Autodesk Inventor part; units mm, degrees
ref_plane "YZ Plane" through (0, 0, 0) normal (1, 0, 0) x (0, 1, 0)
ref_plane "XZ Plane" through (0, 0, 0) normal (0, 1, 0) x (-1, 0, 0)
ref_plane "XY Plane" through (0, 0, 0) normal (0, 0, 1) x (1, 0, 0)
ref_plane "Plano de trabajo1" through (0, 0, 0) normal (0, 0, 1) x (1, 0, 0)
sketch "Boceto1" plane through (0, 0, 0) normal (0, 0, 1) x (1, 0, 0)
  circle A0 centre (18.3423, 0) radius 1.2028
  circle A1 centre (3.6423, 0) radius 1.2028
  circle A2 centre (10.9923, -7.35) radius 1.2028
  circle A3 centre (10.9923, 7.35) radius 1.2028
  circle A4 centre (10.9923, 0) radius 10.9823
  circle A5 centre (10.9923, 0) radius 2.7
  circle A6 centre (10.9923, 0) radius 12.5
  line L0 (10.9923, 0) -> (22.9923, 0)
  line L1 (10.9923, 0) -> (10.9923, 12.5)
  line L2 (10.9923, 12.5) -> (22.9923, 12.5)
  line L3 (10.9923, 0) -> (10.9923, -12.5)
  line L4 (10.9923, -12.5) -> (22.9923, -12.5)
  line L5 (22.9923, -12.5) -> (22.9923, 12.5)
  point P0 (0, 0)
  dimension "d0" = 25
  dimension "d1" = 12
  dimension "d2" = 12
extrude "Extrusión1" add sketch "Boceto1" along normal blind 3 contours L0 A4 L3 A2 A5 A0 | A0 L0 A5 L1 A3 A4 | L0 L5 A6 L3 A4 | A4 L1 A6 L5 L0 | L1 A3 A5 L3 A2 A4 | A4 L3 A6 L1 | L2 L5 A6 | A6 L5 L4
sketch "Boceto2" plane through (22.9923, -12.5, 0) normal (1, 0, 0) x (0, 0, -1)
  line L0 (0, 0) -> (0, 25)
  line L1 (0, 25) -> (-3, 25)
  line L2 (-3, 0) -> (-3, 25)
  line L3 (0, 0) -> (-3, 0)
  point P0 (0, 12.5)
extrude "Extrusión2" add sketch "Boceto2" along normal blind 8
sketch "Boceto3" plane through (0, 0, 0) normal (0, 0, -1) x (-1, 0, 0)
  line L0 (-10.9923, -12.5) -> (-30.9923, -12.5)
  arc A0 (-10.9923, -12.5) -> (-10.9923, 12.5) centre (-10.9923, 0) ccw
  line L1 (-10.9923, 12.5) -> (-30.9923, 12.5)
  line L2 (-30.9923, -12.5) -> (-30.9923, 12.5)
  circle A1 centre (-10.9923, 0) radius 2.7
  circle A2 centre (-10.9923, 7.35) radius 1.2028
  circle A3 centre (-18.3423, 0) radius 1.2028
  circle A4 centre (-3.6423, 0) radius 1.2028
  circle A5 centre (-10.9923, -7.35) radius 1.2028
  line L3 (-30.9923, 12.5) -> (-27.9923, 12.5)
  line L4 (-27.9923, 12.5) -> (-27.9923, -12.5)
  line L5 (-27.9923, -12.5) -> (-30.9923, -12.5)
  line L6 (-30.9923, -12.5) -> (-30.9923, 12.5)
  point P0 (0, 0)
  dimension "d7" = 3
extrude "Extrusión3" add sketch "Boceto3" along normal blind 42 contours L0 L2 L1 L4
sketch "Boceto4" plane through (27.9923, -12.5, 0) normal (-1, 0, 0) x (0, 0, 1)
  line L0 (-42, 0) -> (-42, 25)
  line L1 (0, 25) -> (0, 0)
  line L2 (0, 25) -> (-42, 25)
  line L3 (-42, 0) -> (-42, 25)
  line L4 (0, 0) -> (-42, 0)
  line L5 (-42, 0) -> (-40, 0)
  line L6 (-40, 0) -> (-40, 25)
  line L7 (-40, 25) -> (-42, 25)
  line L8 (-42, 25) -> (-42, 0)
  point P0 (0, 12.5)
  dimension "d10" = 2
extrude "Extrusión4" add sketch "Boceto4" along normal blind 30 contours L0 L2 L6 L4
sketch "Boceto5" plane through (0, 0, -42) normal (0, 0, -1) x (-1, 0, 0)
  line L0 (24.4501, 12.6367) -> (24.5578, -12.3277)
  line L1 (-11.0672, 12.4835) -> (24.4501, 12.6367)
  arc A0 (-11.0672, 12.4835) -> (-10.9596, -12.4809) centre (-11.0134, 0.0013) ccw
  line L2 (-10.9596, -12.4809) -> (24.5578, -12.3277)
  circle A1 centre (-3.6676, 0.2495) radius 1.2028
  circle A2 centre (-11.0134, 0.0013) radius 2.7
  circle A3 centre (-10.7652, -7.3445) radius 1.2028
  circle A4 centre (-11.2616, 7.3471) radius 1.2028
  circle A5 centre (-18.3592, -0.2469) radius 1.2028
  line L3 (-30.9923, 12.5) -> (2.0077, 12.5)
  line L4 (-11.0672, 12.4835) -> (2.0077, 12.5)
  line L5 (2.0391, -12.4248) -> (2.0077, 12.5)
  line L6 (-10.9596, -12.4809) -> (2.0391, -12.4248)
  line L7 (-11.0672, 12.4835) -> (2.0077, 12.5)
  circle A6 centre (-11.0134, 0.0013) radius 12.4823
  line L8 (-10.7652, -7.3445) -> (-10.7652, -14.8497)
  line L9 (-10.7652, -14.8497) -> (6.2045, -14.8497)
  line L10 (6.2045, -14.8497) -> (6.2045, 15.7882)
  line L11 (6.2045, 15.7882) -> (-10.7652, 15.7882)
  line L12 (-10.7652, 15.7882) -> (-11.2616, 7.3471)
  point P0 (0, 0)
  point P1 (-7.2489, 12.5)
  point P2 (-10.991, 12.4836)
  point P3 (-10.9817, -12.481)
  point P4 (-10.9586, 12.5)
  point P5 (6.2045, 12.558)
  point P6 (6.2045, -12.4069)
  point P7 (-10.7652, -12.48)
  point P8 (-10.9595, 12.484)
  point P9 (-10.9595, 12.4837)
  point P10 (-10.9596, 12.4835)
  point P11 (-10.991, 12.4836)
  point P12 (-10.7652, -12.4785)
  point P13 (-11.0672, 12.4835)
extrude "Extrusión5" cut sketch "Boceto5" against normal blind 25 contours L10 L2 L5 L3 L1 | L1 L3 L12 L11 L10 | L10 L9 L8 L2 | L3 L4 L1 | L1 L12 L3 | L2 A6 L4 L5 | A3 | A4 | A1 | A2 | A5
sketch "Boceto8" plane through (10.9923, -12.5, 0) normal (0, -1, 0) x (1, 0, 0)
  line L0 (-0.2271, -40) -> (-0.2271, -42)
  line L1 (20, -42) -> (-0.2271, -42)
  line L2 (20, 3) -> (20, -42)
  line L3 (0, 3) -> (20, 3)
  line L4 (0, 0) -> (0, 3)
  line L5 (0, 0) -> (17, 0)
  line L6 (17, 0) -> (17, -40)
  line L7 (17, -40) -> (-0.2271, -40)
  line L8 (20, -42) -> (20, -19.5)
  line L9 (20, 3) -> (20, -42)
  line L10 (20, -19.5) -> (20, -23.5)
  line L11 (20, -23.5) -> (20, -15.5)
  line L12 (20, -15.5) -> (17, -15.5)
  line L13 (20, -23.5) -> (17, -23.5)
  point P0 (-10.9923, 0)
  dimension "d29" = 22.5
  dimension "d30" = 4
  dimension "d31" = 8
extrude "Extrusión8" add sketch "Boceto8" along normal blind 6 contours L6 L12 L2 L13
ref_plane "Plano de trabajo2" through (-0.8313, -11.6464, -27.56) normal (0.0048, -1, 0) x (1, 0.0048, 0)
sketch "Boceto9" plane through (30.9923, -12.5, 0) normal (1, 0, 0) x (0, 0, -1)
  line L0 (-3, 25) -> (42, 25)
  line L1 (-3, 25) -> (-3, 0)
  line L2 (-3, 0) -> (15.5, 0)
  line L3 (15.5, 0) -> (15.5, -6)
  line L4 (23.5, -6) -> (15.5, -6)
  line L5 (23.5, 0) -> (23.5, -6)
  line L6 (23.5, 0) -> (42, 0)
  line L7 (42, 25) -> (42, 0)
  line L8 (23.5, 0) -> (23.5, 25)
  line L9 (23.5, 25) -> (23.5, 31)
  line L10 (23.5, 31) -> (15.5, 31)
  line L11 (15.5, 31) -> (15.5, 25)
  point P0 (0, 12.5)
  dimension "d34" = 6
extrude "Extrusión9" add sketch "Boceto9" against normal blind 3 contours L11 L10 L9 L0
sketch "Boceto10" plane through (27.9923, -12.5, 0) normal (-1, 0, 0) x (0, 0, 1)
  line L0 (-40, 25) -> (-40, 0)
  line L1 (-23.5, 0) -> (-40, 0)
  line L2 (-23.5, 0) -> (-23.5, -6)
  line L3 (-15.5, -6) -> (-23.5, -6)
  line L4 (-15.5, 0) -> (-15.5, -6)
  line L5 (0, 0) -> (-15.5, 0)
  line L6 (0, 25) -> (0, 0)
  line L7 (0, 25) -> (-15.5, 25)
  line L8 (-15.5, 25) -> (-15.5, 31)
  line L9 (-15.5, 31) -> (-23.5, 31)
  line L10 (-23.5, 31) -> (-23.5, 25)
  line L11 (-23.5, 25) -> (-40, 25)
  line L12 (-15.5, -3) -> (-19.5, -3)
  line L13 (-19.5, -3) -> (-19.5, 28)
  circle A0 centre (-19.5, -3) radius 1.25
  circle A1 centre (-19.5, 28) radius 1.25
  point P0 (0, 12.5)
  dimension "d37" = 2.5
  dimension "d38" = 2.5
extrude "Extrusión10" cut sketch "Boceto10" against normal blind 3 contours A1 | A0 L13 L12 | L12 L13 A0
sketch "Boceto11" plane through (27.9923, -12.5, 0) normal (-1, 0, 0) x (0, 0, 1)
  line L0 (-42, 25) -> (-42, 0)
  line L1 (-42, 25) -> (-42, 12.5)
  line L2 (-42, 12.5) -> (-19.5, 12.5)
  line L3 (3, 13.7028) -> (3, 11.2972)
  line L4 (-19.5, 12.5) -> (-19.5, 25)
  point P0 (0, 12.5)
  dimension "d41" = 12.5
  dimension "d42" = 22.5
sketch "Boceto12" plane through (27.9923, -12.5, -40) normal (0, 0, 1) x (1, 0, 0)
  circle A0 centre (-16.9789, 12.5013) radius 5.6
  circle A1 centre (-16.9789, 12.5013) radius 5.6
  circle A2 centre (-16.9789, 12.5013) radius 2.7
  point P0 (-27.9923, 12.5)
extrude "Extrusión11" cut sketch "Boceto12" against normal blind 10
sketch "Boceto13" plane through (27.9923, -12.5, -40) normal (0, 0, 1) x (1, 0, 0)
  circle A0 centre (-16.9789, 12.5013) radius 5.6
  line L0 (-17.0337, 25) -> (-17.0328, 24.9835)
  arc A1 (-17.0328, 24.9835) -> (-17.2271, 0.0215) centre (-16.9789, 12.5013) ccw
  line L1 (-17.2271, 0.0215) -> (-17.2271, 0)
  line L2 (0, 0) -> (-17.2271, 0)
  line L3 (0, 25) -> (0, 0)
  line L4 (0, 25) -> (-17.0337, 25)
  circle A2 centre (-9.6331, 12.2531) radius 1.2028
  circle A3 centre (-16.7307, 19.8471) radius 1.2028
  circle A4 centre (-17.2271, 5.1555) radius 1.2028
  circle A5 centre (-24.3247, 12.7495) radius 1.2028
  point P0 (-27.9923, 12.5)
extrude "Extrusión12" add sketch "Boceto13" along normal blind 6
sketch "Boceto15" plane through (27.9923, -12.5, -34) normal (0, 0, 1) x (1, 0, 0)
  line L0 (-17.0337, 25) -> (-17.0328, 24.9835)
  arc A0 (-17.0328, 24.9835) -> (-17.2271, 0.0215) centre (-16.9789, 12.5013) ccw
  line L1 (-17.2271, 0.0215) -> (-17.2271, 0)
  line L2 (-17.2271, 0) -> (0, 0)
  line L3 (0, 25) -> (0, 0)
  line L4 (0, 25) -> (-17.0337, 25)
  circle A1 centre (-9.6331, 12.2531) radius 1.2028
  circle A2 centre (-24.3247, 12.7495) radius 1.2028
  circle A3 centre (-17.2271, 5.1555) radius 1.2028
  circle A4 centre (-16.7307, 19.8471) radius 1.2028
  circle A5 centre (-16.9789, 12.5013) radius 5.6
  point P0 (-27.9923, 12.5)
extrude "Extrusión14" cut sketch "Boceto15" against normal blind 3
sketch "Boceto16" plane through (0, 0, -42) normal (0, 0, -1) x (-1, 0, 0)
  circle A0 centre (-11.0134, 0.0013) radius 5.6
  line L0 (-10.9596, 12.4835) -> (-10.9586, 12.5)
  line L1 (-30.9923, 12.5) -> (-10.9586, 12.5)
  line L2 (-30.9923, 12.5) -> (-30.9923, -12.5)
  line L3 (-30.9923, -12.5) -> (-10.7652, -12.5)
  line L4 (-10.7652, -12.5) -> (-10.7652, -12.4785)
  arc A1 (-10.7652, -12.4785) -> (-10.9596, 12.4835) centre (-11.0134, 0.0013) ccw
  circle A2 centre (-3.6676, 0.2495) radius 1.2028
  circle A3 centre (-10.7652, -7.3445) radius 1.2028
  circle A4 centre (-11.2616, 7.3471) radius 1.2028
  circle A5 centre (-18.3592, -0.2469) radius 1.2028
  point P0 (0, 0)
extrude "Extrusión15" cut sketch "Boceto16" against normal blind 2
properties part number "UnionCuerpo"
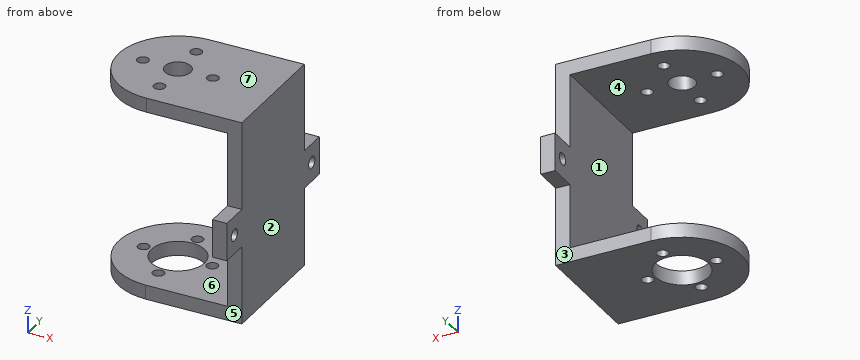
Geometry check sheet. Reference: the model listing, model coordinates, mm. Face numbers are marked on the shaded views. A direction names the side the tool comes from. Give positions to 0.01 mm unless a question says otherwise; leave off trailing zeros. Order: outer loops, then holes, each group sorted by start corner. A loop starts at its lowest first (then second) coordinate and runs counter-clockwise, first axis right, second up.
1) Gauge pin test, flat ends, axial feed: pin 1 (2.5 mm diameter, centred on x = 30, y = -14.5, fed in from +Z); pin 2 (15 mm diameter, centred on x = 22.5, z = -4.5, fed in from -Y); pin 3 (18.5 mm diameter, centred on y = 7, z = -11, fed in from -X); pin 4 (4 mm diameter, centred on x = 10.99, y = 7.35, fed in from +Z). Record the tip position at first contact, or that the pin passes through.
Results are:
pin 1: stops at z = -15.5
pin 2: stops at y = -12.5
pin 3: stops at x = 27.99
pin 4: stops at z = 3
2) Cross-section at A-A (y = -15.5). Record the boundary of the cut face in (x, z), then the cut area to 3 significant figures.
Results are:
outline: (27.99, -23.5) - (30.99, -23.5) - (30.99, -20.75) - (27.99, -20.75) - close; (27.99, -18.25) - (30.99, -18.25) - (30.99, -15.5) - (27.99, -15.5) - close
area: 16.5 mm2
3) Cross-section at D-D (y = -4). Record the boundary of the cut face in (x, z), then the cut area to 3 significant figures.
Results are:
outline: (-0.85, 0) - (27.99, 0) - (27.99, -37) - (14.93, -37) - (14.93, -40) - (30.99, -40) - (30.99, 3) - (-0.85, 3) - close; (-0.81, -40) - (7.1, -40) - (7.1, -37) - (-0.81, -37) - close
area: 278 mm2
4) Cross-section at C-C (z = -19.5). Record the boundary of the cut face in (x, y).
Results are:
outline: (27.99, -18.5) - (30.99, -18.5) - (30.99, -16.75) - (27.99, -16.75) - close; (27.99, -14.25) - (30.99, -14.25) - (30.99, 14.25) - (27.99, 14.25) - close; (27.99, 16.75) - (30.99, 16.75) - (30.99, 18.5) - (27.99, 18.5) - close
5) Material ranges on probe 1 along Y at (x, z) = (29.7, -19.5); probe 2 along Z at (x, y) = (12.5, -6); probe 3 along Z at (x, y) = (29.25, 15.5), recorded low to high.
Results are:
probe 1: y = -18.5 to -16.75, -14.25 to 14.25, 16.75 to 18.5
probe 2: z = -40 to -37, 0 to 3
probe 3: z = -23.5 to -20.75, -18.25 to -15.5
6) Draft check along Z on the marked faces 4, 5, 6 and 7. Enter one of: released by +Z, released by -Z, zero draft, split by the parting line, or undercut.
Results are:
face 4: undercut
face 5: zero draft
face 6: undercut
face 7: released by +Z
7) Cross-section at B-B (x = 23). Record the boundary of the cut face in (y, z).
Results are:
outline: (-12.5, -40) - (12.5, -40) - (12.5, -37) - (-12.5, -37) - close; (-12.5, 0) - (12.5, 0) - (12.5, 3) - (-12.5, 3) - close
8) Tool access check on the marked faces 1, 2 and 3. Record the directions out of +Z, -Z, +X, -X, +Y, -Y that give a thin tool (end or side, any length) a straight path to the whole face; none if there is none.
Results are:
face 1: -X, +Y, -Y
face 2: +Z, -Z, +X, +Y, -Y
face 3: -Z, +X, -X, +Y
